Read the model definition and answer for the solid it produces. Units are mm, in the model's axes. A direction names the side the tool comes from. Round coordinates to 2 decimals unless told otherwise and drop trailing zeros. Write each loop counter-clockwise with the first axis right and the second up, starting at its lowest first coordinate (ties: lowest second). Pieces come first, ordered by that corner, then holes. Notation, with made-up numbers: (42, -7) - (59, -7) arc R15 cw to (59, 1) - close; hole circle Ø2 at (-16.75, -3.5). An arc over 180 degrees is marked (long way). Answer as CSV lines item,"result". Start each with the question number.
1) Which of the six approach directions +Z, -Z, +X, -X, +Y, -Y give full straight-line access (tool end or side, diameter ignored) to faces 5 (the flat face through (-51, 0, 13)), 6 (the flat face through (-1, 188, 2))?
2) Consider line 1 along X through (y, z) = (130.5, -21.5); line 2 along Z through (x, y) = (-115, 110.5); line 3 along Z through (x, y) = (42.5, 171.5). Determine where each line is inside the solid, lowest interval first.
3) Find section A-A on y = 48.5. Determine the outline of the cut face in (x, z).
4) For a pull along X with two mould halves and no side action, classify faces 1 (the flat face through (136, 93, -156)), 2 (the flat face through (224, 99, -2)), 3 (the flat face through (62, 95, 80)), 4 (the flat face through (-3, 99, -168)) as +X half, -X half, draft (parallel to the pull), parting line (faces both ways), or undercut.
5) Find section B-B on x = 26. Determine the outline of the cut face in (y, z).
6) Find section D-D on x = 169.5. Determine the outline of the cut face in (y, z).
7) Find section C-C on z = -25. Determine the outline of the cut face in (x, y).
from build123d import *

# Parameters (mm, degrees)
F0_W     = 448
F0_H     = 336
F1_DEPTH = 200
F2_T     = -12
F3_W     = 150
F3_H     = 12
F4_DEPTH = 188


with BuildPart() as f1:
    # F0 (on Front) → F1 (new body)
    with BuildSketch(Plane.XZ):
        Rectangle(F0_W, F0_H)
    extrude(amount=-F1_DEPTH)

    # F2
    f2_openings = [f1.faces().sort_by_distance(p)[0] for p in [
        (0, 0, 0),
    ]]
    offset(amount=F2_T, openings=f2_openings)

    # F3 (on face) → F4 (join)
    with BuildSketch(Plane.XZ.offset(-188)):
        with Locations((-137, 0)):
            Rectangle(F3_W, F3_H)
        Polygon((-50, 156), (-62, 156), (-62, 6), (-62, -6), (-62, -156), (-50, -156), align=None)
        Polygon((62, 156), (50, 156), (50, -156), (62, -156), (62, -6), (62, 6), align=None)
        with Locations((137, 0)):
            Rectangle(F3_W, F3_H)
    extrude(amount=F4_DEPTH)


solid = f1.part
Check values:
1,face 5,"+Z, -Z, +X, -X, -Y"
1,face 6,"-Y"
2,line 1,"x = -224 to -212, -62 to -50, 50 to 62, 212 to 224"
2,line 2,"z = -168 to -156, -6 to 6, 156 to 168"
2,line 3,"z = -168 to -156, 156 to 168"
3,outline,"(-224, -168) - (224, -168) - (224, 168) - (-224, 168) - close; hole (-212, -156) - (-62, -156) - (-62, -6) - (-212, -6) - close; hole (-212, 6) - (-62, 6) - (-62, 156) - (-212, 156) - close; hole (-50, -156) - (50, -156) - (50, 156) - (-50, 156) - close; hole (62, -156) - (212, -156) - (212, -6) - (62, -6) - close; hole (62, 6) - (212, 6) - (212, 156) - (62, 156) - close"
4,face 1,"undercut"
4,face 2,"+X half"
4,face 3,"undercut"
4,face 4,"draft"
5,outline,"(0, -168) - (200, -168) - (200, 168) - (0, 168) - (0, 156) - (188, 156) - (188, -156) - (0, -156) - close"
6,outline,"(0, -168) - (200, -168) - (200, 168) - (0, 168) - (0, 156) - (188, 156) - (188, 6) - (0, 6) - (0, -6) - (188, -6) - (188, -156) - (0, -156) - close"
7,outline,"(-224, 0) - (-212, 0) - (-212, 188) - (-62, 188) - (-62, 0) - (-50, 0) - (-50, 188) - (50, 188) - (50, 0) - (62, 0) - (62, 188) - (212, 188) - (212, 0) - (224, 0) - (224, 200) - (-224, 200) - close"
